Verification items for this drawing (mm, ordinates from the low corner). Coordinates: 2 decimals unless noted, no trailing zeros. Loops run counter-clockwise (first coordinate to the right, second up) from the corner with the lowest first, then second, coordinate; pieces in that order, holes last. Notation, with made-up numbers: (-28.5, 37.5) - (-9.5, 37.5) arc R12 ccw to (-9.5, 58.5) - close; hole circle Ø10 at (-22.5, 49). An arc over 180 degrees is marked (long way). One line per item, written item: value. Start each with the question number.
(1) Thickness scan on probe 1 along Y at (x, z) = (15, 3.5); probe 2 along X at (y, z) = (30.5, 2.75); probe 3 along X at (y, z) = (12, 5.75). Record the ranges inside material, lowest first. Write a range as [from, to].
(2) Draft check along X on the marked faces 1 and 2. Enter one of: +X half, -X half, draft (parallel to the pull), parting line (faces both ways), or undercut.
(3) Section check B-B (z = 3). Record the boundary of the cut face in (x, y).
(4) Section check A-A (y = 17.5). Record the boundary of the cut face in (x, z), plus the area to 3 significant figures.
(5) Section check C-C (x = 15). Record the boundary of the cut face in (y, z).
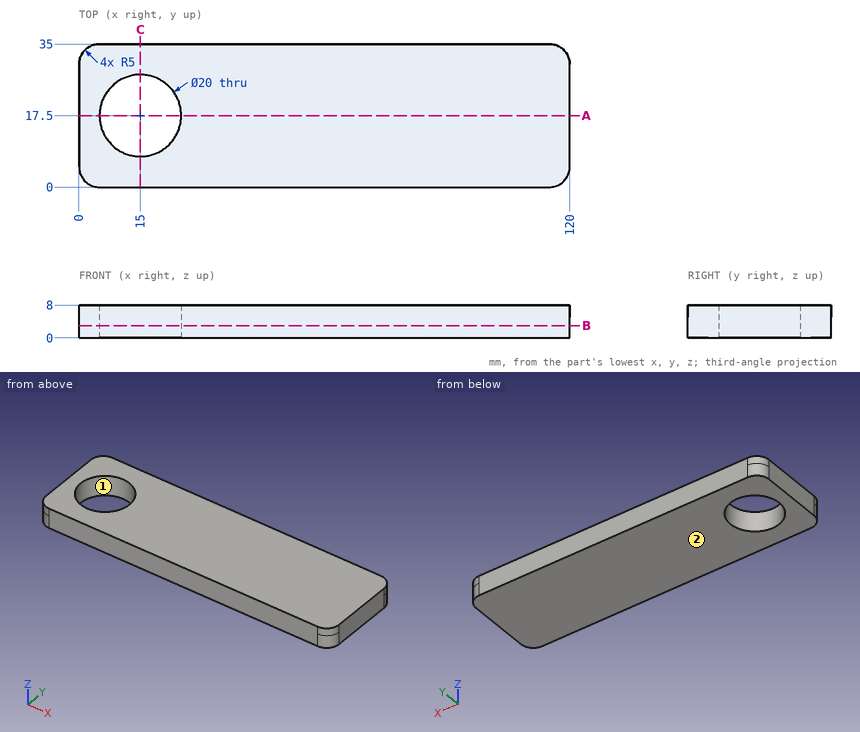
Responses:
1. probe 1: y = [0, 7.5], [27.5, 35]
1. probe 2: x = [0.03, 119.97]
1. probe 3: x = [0, 6.65], [23.35, 120]
2. face 1: undercut
2. face 2: draft
3. outline: (0, 5) arc R5 ccw to (5, 0) - (115, 0) arc R5 ccw to (120, 5) - (120, 30) arc R5 ccw to (115, 35) - (5, 35) arc R5 ccw to (0, 30) - close; hole circle Ø20 at (15, 17.5)
4. outline: (0, 0) - (5, 0) - (5, 8) - (0, 8) - close; (25, 0) - (120, 0) - (120, 8) - (25, 8) - close
4. area: 800 mm²
5. outline: (0, 0) - (7.5, 0) - (7.5, 8) - (0, 8) - close; (27.5, 0) - (35, 0) - (35, 8) - (27.5, 8) - close
